Source: CAD feature listing. Evaluate the final solid. Frame: model axes, mm. Face numbers are marked on the shaded views. A direction names the side the tool comes from. Round coordinates to 2 decimals unless told otherwise and drop trailing zeros. Order: outer loops, then holes, each group sorted by start corner. A loop starts at its lowest first (then second) coordinate and runs counter-clockwise, first axis right, second up. Notation, with made-up numbers: (-18, 87) - (-6, 87) arc R11 ccw to (-6, 94) - close; hole circle Ø5 at (-27.75, -5.5). An arc over 180 degrees is marked (long way). Use one line per item in the form item = value. Start each with the question number.
Q1. Cut plane B-B, the plane z = -6.35. Return the cut outline in (x, y) (3 decimals).
Q2. Cut plane C-C, the plane x = 8. Return the cut outline in (y, z) (3 decimals).
Q3. Cut plane D-D, the plane z = 25. Return the cut outline in (x, y) (3 decimals), and give its area (3 significant figures).
Q4. Cut plane A-A, the plane y = 50.8. Return the cut outline in (x, z) (3 decimals).
Q5. Ray query, line 1 (Y direction, x = 28, z = -6); line 2 (Z direction, x = 20.5, y = 50.8) (3 decimals); line 3 (X direction, y = -1, z = 51). Return the intervals inside material, ascending. Write a range as [from, to].
Q6. Set-up query: the marked faces 4, 5, 6, 7 and 8. Return all of +Z, -Z, +X, -X, +Y, -Y with unobstructed straight access to the full face (end or side cutting, diameter ignored); none if empty.
Q7. Pin query (flat end, axial travel): pin 1 Ø6 at (y, z) = (23.5, 47.5) entering from +X; pin 2 Ø6 at (x, z) = (25, 43.5) entering from +Y; pin 3 Ø7.5 at (y, z) = (50.8, -6.35) entering from -X; pin 4 Ø10 at (x, z) = (17, -4) entering from -Y. Return the tip coordinate at first contact, or that it passes through.
Q8. Draft query along Z for the marked faces 1, 2 and 3. Return one class per face: released by +Z, released by -Z, zero draft, split by the parting line, or undercut.
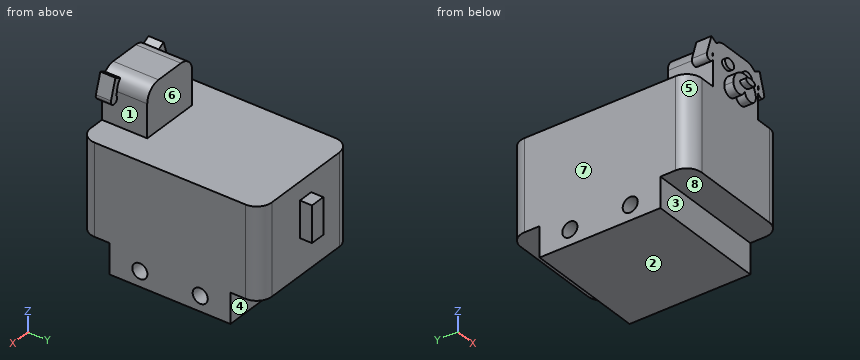
from build123d import *

# Parameters (mm, degrees)
F1_DEPTH  = 38.1
F3_W      = 50.8
F3_H      = 12.7
F3_R      = 3.175
F4_DEPTH  = 50.8
F6_DEPTH  = 19.05
F7_DEPTH  = 3.81
F9_DEPTH  = 2.54
F11_DEPTH = 6.35
F12_DEPTH = 1.27
F13_W     = 6.35
F13_H     = 15.24
F14_DEPTH = 5.08


with BuildPart() as f1:
    # F0 (on Top) → F1 (new body)
    with BuildSketch(Plane.XY):
        with BuildLine():
            Line((0, 69.85), (0, 6.35))
            ThreePointArc((0, 6.35), (1.8598719395, 1.8598719395), (6.35, 0))
            Line((6.35, 0), (44.45, 0))
            ThreePointArc((44.45, 0), (48.9401280605, 1.8598719395), (50.8, 6.35))
            Line((50.8, 6.35), (50.8, 69.85))
            ThreePointArc((50.8, 69.85), (48.9401280605, 74.3401280605), (44.45, 76.2))
            Line((44.45, 76.2), (6.35, 76.2))
            ThreePointArc((6.35, 76.2), (1.8598719395, 74.3401280605), (0, 69.85))
        make_face()
    extrude(amount=F1_DEPTH)

    # F3 (on face) → F4 (join, through all)
    with BuildSketch(Plane(origin=(0, 0, 0), x_dir=(0, -1, 0), z_dir=(-1, 0, 0))):
        with Locations((-38.1, -6.35)):
            Rectangle(F3_W, F3_H)
        with Locations((-50.8, -6.35)):
            Circle(F3_R, mode=Mode.SUBTRACT)
        with Locations((-25.4, -6.35)):
            Circle(F3_R, mode=Mode.SUBTRACT)
    extrude(amount=-F4_DEPTH)

    # F5 (on face) → F6 (join)
    with BuildSketch(Plane.XZ):
        with BuildLine():
            Line((12.7, 52.07), (12.7, 38.1))
            Line((12.7, 38.1), (38.1, 38.1))
            Line((38.1, 38.1), (38.1, 52.07))
            ThreePointArc((38.1, 52.07), (36.2401280605, 56.5601280605), (31.75, 58.42))
            Line((31.75, 58.42), (19.05, 58.42))
            ThreePointArc((19.05, 58.42), (14.5598719395, 56.5601280605), (12.7, 52.07))
        make_face()
        with BuildLine():
            ThreePointArc((19.05, 41.91), (20.9098719395, 46.4001280605), (25.4, 48.26))
            ThreePointArc((25.4, 48.26), (29.8901280605, 46.4001280605), (31.75, 41.91))
            ThreePointArc((31.75, 41.91), (28.575, 38.735), (25.4, 41.91))
            ThreePointArc((25.4, 41.91), (22.225, 38.735), (19.05, 41.91))
        make_face(mode=Mode.SUBTRACT)
        with BuildLine():
            ThreePointArc((31.75, 41.91), (29.8901280605, 46.4001280605), (25.4, 48.26))
            ThreePointArc((25.4, 48.26), (20.9098719395, 46.4001280605), (19.05, 41.91))
            ThreePointArc((19.05, 41.91), (22.225, 38.735), (25.4, 41.91))
            ThreePointArc((25.4, 41.91), (28.575, 38.735), (31.75, 41.91))
        make_face()
    extrude(amount=-F6_DEPTH)

    # F5 (on face) → F7 (join)
    with BuildSketch(Plane.XZ):
        with BuildLine():
            ThreePointArc((31.75, 41.91), (29.8901280605, 46.4001280605), (25.4, 48.26))
            ThreePointArc((25.4, 48.26), (20.9098719395, 46.4001280605), (19.05, 41.91))
            ThreePointArc((19.05, 41.91), (22.225, 38.735), (25.4, 41.91))
            ThreePointArc((25.4, 41.91), (28.575, 38.735), (31.75, 41.91))
        make_face()
    extrude(amount=F7_DEPTH)

    # F8 (on face) → F9 (join)
    with BuildSketch(Plane.XZ.offset(3.81)):
        with BuildLine():
            add(Edge.make_bspline(
                [(27.94, 44.1034744838), (27.94, 46.3031790094), (24.13, 45.2033267466), (20.32, 44.1034744838), (24.13, 43.003622221), (27.94, 41.9037699582), (27.94, 44.1034744838)],
                knots=[0, 0, 0, 2.0943951024, 2.0943951024, 4.1887902048, 4.1887902048, 6.2831853072, 6.2831853072, 6.2831853072], degree=2, weights=[1, 0.5, 1, 0.5, 1, 0.5, 1]))
        make_face()
    extrude(amount=F9_DEPTH)

    # F10 (on face) → F11 (join)
    with BuildSketch(Plane.XZ):
        with BuildLine():
            Line((17.78, 50.8), (22.86, 50.8))
            add(Edge.make_bspline(
                [(22.86, 50.8), (22.86, 52.832), (20.32, 52.832), (17.78, 52.832), (17.78, 50.8)],
                knots=[0, 0, 0, 1.5707963268, 1.5707963268, 3.1415926536, 3.1415926536, 3.1415926536], degree=2, weights=[1, 0.7071067812, 1, 0.7071067812, 1]))
        make_face()
        with BuildLine():
            add(Edge.make_bspline(
                [(17.78, 50.8), (17.78, 48.768), (20.32, 48.768), (22.86, 48.768), (22.86, 50.8)],
                knots=[3.1415926536, 3.1415926536, 3.1415926536, 4.7123889804, 4.7123889804, 6.2831853072, 6.2831853072, 6.2831853072], degree=2, weights=[1, 0.7071067812, 1, 0.7071067812, 1]))
            Line((22.86, 50.8), (17.78, 50.8))
        make_face()
        with BuildLine():
            add(Edge.make_bspline(
                [(27.94, 50.8), (27.94, 48.768), (30.48, 48.768), (33.02, 48.768), (33.02, 50.8)],
                knots=[3.1415926536, 3.1415926536, 3.1415926536, 4.7123889804, 4.7123889804, 6.2831853072, 6.2831853072, 6.2831853072], degree=2, weights=[1, 0.7071067812, 1, 0.7071067812, 1]))
            Line((33.02, 50.8), (27.94, 50.8))
        make_face()
        with BuildLine():
            Line((27.94, 50.8), (33.02, 50.8))
            add(Edge.make_bspline(
                [(33.02, 50.8), (33.02, 52.832), (30.48, 52.832), (27.94, 52.832), (27.94, 50.8)],
                knots=[0, 0, 0, 1.5707963268, 1.5707963268, 3.1415926536, 3.1415926536, 3.1415926536], degree=2, weights=[1, 0.7071067812, 1, 0.7071067812, 1]))
        make_face()
        with BuildLine():
            ThreePointArc((36.2401280605, 56.5601280605), (37.6166350314, 54.5000397955), (38.1, 52.07))
            Line((38.1, 52.07), (38.5869643704, 50.8))
            ThreePointArc((38.5869643704, 50.8), (38.2785524575, 50.3900976738), (38.1, 49.9092059552))
            Line((38.1, 49.9092059552), (38.1, 49.1652853166))
            ThreePointArc((38.1, 49.1652853166), (40.2931830208, 47.8183243314), (41.5339241122, 50.0733004294))
            Line((41.5339241122, 50.0733004294), (39.0068086574, 58.0652721184))
            Line((39.0068086574, 58.0652721184), (36.2401280605, 56.5601280605))
        make_face()
        with BuildLine():
            Line((12.2130356296, 50.8), (12.7, 52.07))
            ThreePointArc((12.7, 52.07), (13.1833649686, 54.5000397955), (14.5598719395, 56.5601280605))
            Line((14.5598719395, 56.5601280605), (11.7931913426, 58.0652721184))
            Line((11.7931913426, 58.0652721184), (9.2660758878, 50.0733004294))
            ThreePointArc((9.2660758878, 50.0733004294), (10.5068169792, 47.8183243314), (12.7, 49.1652853166))
            Line((12.7, 49.1652853166), (12.7, 49.9092059552))
            ThreePointArc((12.7, 49.9092059552), (12.5214475425, 50.3900976738), (12.2130356296, 50.8))
        make_face()
    extrude(amount=-F11_DEPTH)

    # F10 (on face) → F12 (join)
    with BuildSketch(Plane.XZ):
        with BuildLine():
            Line((17.78, 50.8), (22.86, 50.8))
            add(Edge.make_bspline(
                [(22.86, 50.8), (22.86, 52.832), (20.32, 52.832), (17.78, 52.832), (17.78, 50.8)],
                knots=[0, 0, 0, 1.5707963268, 1.5707963268, 3.1415926536, 3.1415926536, 3.1415926536], degree=2, weights=[1, 0.7071067812, 1, 0.7071067812, 1]))
        make_face()
        with BuildLine():
            add(Edge.make_bspline(
                [(17.78, 50.8), (17.78, 48.768), (20.32, 48.768), (22.86, 48.768), (22.86, 50.8)],
                knots=[3.1415926536, 3.1415926536, 3.1415926536, 4.7123889804, 4.7123889804, 6.2831853072, 6.2831853072, 6.2831853072], degree=2, weights=[1, 0.7071067812, 1, 0.7071067812, 1]))
            Line((22.86, 50.8), (17.78, 50.8))
        make_face()
        with BuildLine():
            Line((27.94, 50.8), (33.02, 50.8))
            add(Edge.make_bspline(
                [(33.02, 50.8), (33.02, 52.832), (30.48, 52.832), (27.94, 52.832), (27.94, 50.8)],
                knots=[0, 0, 0, 1.5707963268, 1.5707963268, 3.1415926536, 3.1415926536, 3.1415926536], degree=2, weights=[1, 0.7071067812, 1, 0.7071067812, 1]))
        make_face()
        with BuildLine():
            add(Edge.make_bspline(
                [(27.94, 50.8), (27.94, 48.768), (30.48, 48.768), (33.02, 48.768), (33.02, 50.8)],
                knots=[3.1415926536, 3.1415926536, 3.1415926536, 4.7123889804, 4.7123889804, 6.2831853072, 6.2831853072, 6.2831853072], degree=2, weights=[1, 0.7071067812, 1, 0.7071067812, 1]))
            Line((33.02, 50.8), (27.94, 50.8))
        make_face()
    extrude(amount=F12_DEPTH)

    # F13 (on face) → F14 (join)
    with BuildSketch(Plane(origin=(0, 76.2, 0), x_dir=(-1, 0, 0), z_dir=(0, 1, 0))):
        with Locations((-25.4, 22.86)):
            Rectangle(F13_W, F13_H)
    extrude(amount=F14_DEPTH)


solid = f1.part
Completed:
q1.outline = (0, 12.7) - (50.8, 12.7) - (50.8, 22.225) - (0, 22.225) - close; (0, 28.575) - (50.8, 28.575) - (50.8, 47.625) - (0, 47.625) - close; (0, 53.975) - (50.8, 53.975) - (50.8, 63.5) - (0, 63.5) - close
q2.outline = (0, 0) - (12.7, 0) - (12.7, -12.7) - (63.5, -12.7) - (63.5, 0) - (76.2, 0) - (76.2, 38.1) - (0, 38.1) - close; hole circle Ø6.35 at (25.4, -6.35); hole circle Ø6.35 at (50.8, -6.35)
q3.outline = (0, 6.35) arc R6.35 ccw to (6.35, 0) - (44.45, 0) arc R6.35 ccw to (50.8, 6.35) - (50.8, 69.85) arc R6.35 ccw to (44.45, 76.2) - (28.575, 76.2) - (28.575, 81.28) - (22.225, 81.28) - (22.225, 76.2) - (6.35, 76.2) arc R6.35 ccw to (0, 69.85) - close
q3.area = 3,870 mm2
q4.outline = (0, -12.7) - (50.8, -12.7) - (50.8, -9.525) - (0, -9.525) - close; (0, -3.175) - (50.8, -3.175) - (50.8, 38.1) - (0, 38.1) - close
q5.line_1 = [12.7, 22.24], [28.56, 47.64], [53.96, 63.5]
q5.line_2 = [-12.7, -9.525], [-3.175, 38.1]
q5.line_3 = [17.79, 22.85], [27.95, 33.01]
q6.face_4 = -Z, +X, -X, +Y
q6.face_5 = +Z, -Z, -X, -Y
q6.face_6 = +Z, +X, -X, +Y
q6.face_7 = +Z, -Z, -X, +Y, -Y
q6.face_8 = -Z, +X, -X, -Y
q7.pin_1 = through
q7.pin_2 = 19.05
q7.pin_3 = 0
q7.pin_4 = 0
q8.face_1 = undercut
q8.face_2 = released by -Z
q8.face_3 = zero draft
